Study the drawing (mm; zero at the part's minimum x, y, z) and answer. A direction names the side the tool comes from. Round coordinates to 2 decimals unless told otherwise and drop trailing zeros. Write each loop counter-clockwise with the first axis right and the second up, starting at its lowest first coordinate (ties: lowest second). Pieces come first, ordered by that corner, then holes.
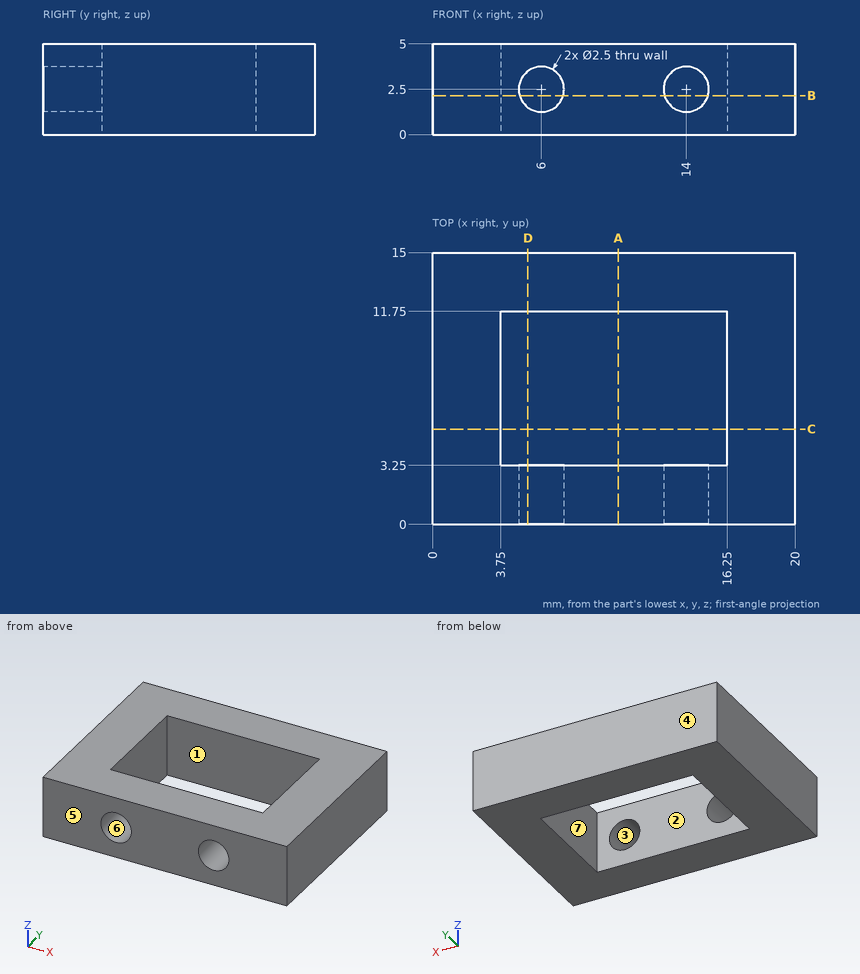
Q1. Find section C-C (y = 5.25). Determine the outline of the cut face in (x, z), plus the area to 3 significant figures.
Q2. Find the intervals of material crossed by L1, parallel to Y at x = 9.5, z = 1.9; L2, parallel to Z at x = 14, y = 2.05; L3, parallel to X at y = 10.5, z = 3.8, in increasing order.
Q3. Find section D-D (x = 5.25). Determine the outline of the cut face in (y, z), plus the area to 3 significant figures.
Q4. Find section A-A (x = 10.25). Determine the outline of the cut face in (y, z).
Q5. The mould has two halves that part along Y. Classify the marked faces 1, 2, 3 and 4: +Y half, -Y half, draft (parallel to the pull), parting line (faces both ways), or undercut.
Q6. Given pin 1 (1 mm diameter, centred on y = 12.5, z = 3.5, fed in from -X), flat-ended and moving along its own axis, determine where the tip first touches the part or whether it passes through.
Q7. Find section B-B (z = 2.15). Determine the outline of the cut face in (x, y), plus the area to 3 significant figures.
Q8. A tool of negligible diameter and unlimited length cuts with its end or side. For the marked faces 5, 6 and 7, from which of +Z, -Z, +X, -X, +Y, -Y can it reach the whole face along a straight path? Write none if from no direction.
Report:
1. outline: (0, 0) - (3.75, 0) - (3.75, 5) - (0, 5) - close; (16.25, 0) - (20, 0) - (20, 5) - (16.25, 5) - close
1. area: 37.5 mm2
2. L1: y = 0 to 3.25, 11.75 to 15
2. L2: z = 0 to 1.25, 3.75 to 5
2. L3: x = 0 to 3.75, 16.25 to 20
3. outline: (0, 0) - (3.25, 0) - (3.25, 1.5) - (0, 1.5) - close; (0, 3.5) - (3.25, 3.5) - (3.25, 5) - (0, 5) - close; (11.75, 0) - (15, 0) - (15, 5) - (11.75, 5) - close
3. area: 26.0 mm2
4. outline: (0, 0) - (3.25, 0) - (3.25, 5) - (0, 5) - close; (11.75, 0) - (15, 0) - (15, 5) - (11.75, 5) - close
5. face 1: undercut
5. face 2: undercut
5. face 3: draft
5. face 4: +Y half
6. pin 1: stops at x = 0
7. outline: (0, 0) - (4.8, 0) - (4.8, 3.25) - (3.75, 3.25) - (3.75, 11.75) - (16.25, 11.75) - (16.25, 3.25) - (15.2, 3.25) - (15.2, 0) - (20, 0) - (20, 15) - (0, 15) - close; (7.2, 0) - (12.8, 0) - (12.8, 3.25) - (7.2, 3.25) - close
7. area: 178 mm2
8. face 5: +Z, -Z, +X, -X, -Y
8. face 6: -Y
8. face 7: +Z, -Z
